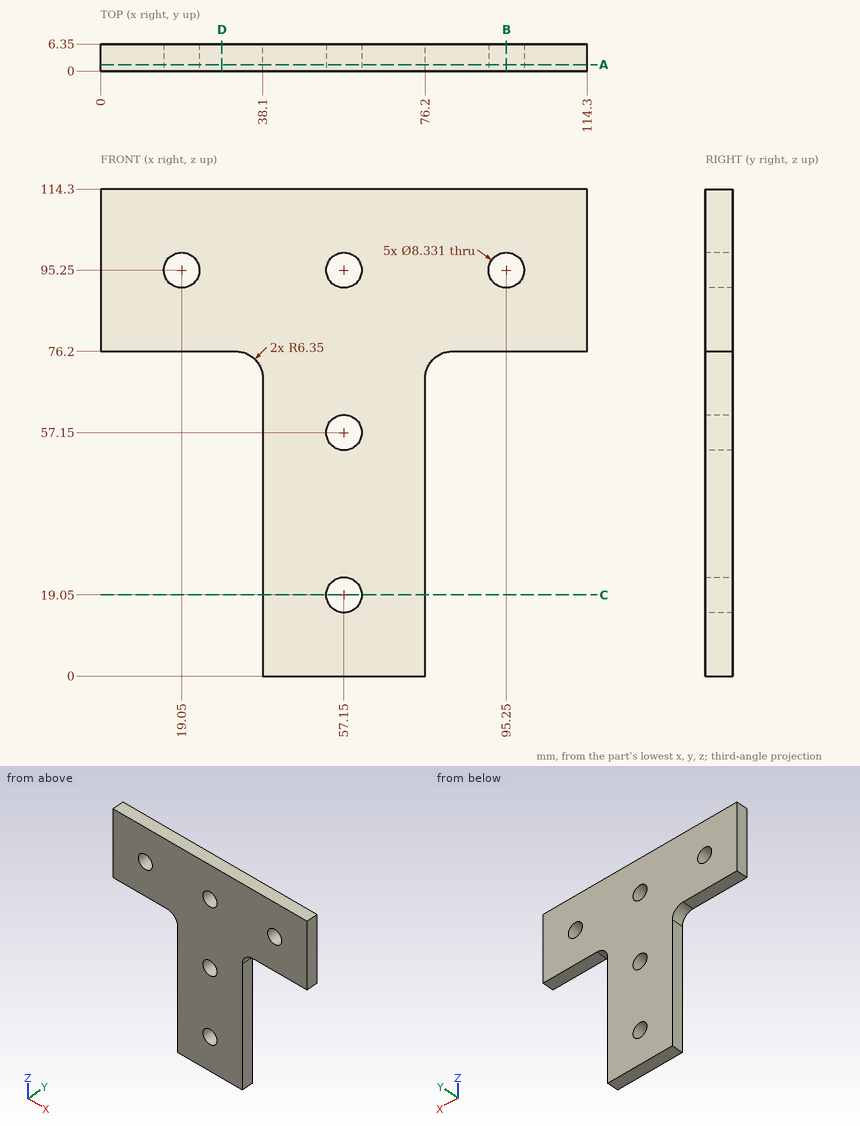
Geometry: see drawing. Coordinates: mm, zero at the bounding-box minimum. Give positions to 0.01 mm unless a question says otherwise; leave off trailing zeros. Order: outer loops, then holes, each group sorted by start corner. A loop starts at its lowest first (then second) coordinate and runs counter-clockwise, first axis right, second up. Notation, with made-up numbers: M 85,68 L 125,68 A36 cw 125,107 Z; hole C -8.5,88.5 d3. An arc over 180 degrees is marked long. Answer as a JSON object with one key per item and string values.
1. First-contact query: P1, Ø6.5, axis at x = 57.15, z = 19.05, coming from the +Y side; P2, Ø3, axis at y = 4.5, z = 51.5, coming from the +X side; P3, Ø3, axis at x = 74, y = 5.5, coming from the -Z side; P4, Ø2, axis at y = 1, z = 38.5, coming from the -X side. Flat tips, straight axial feed; report the tip coordinate or a pass-through.
Result sheet:
{"P1": "through", "P2": "x = 76.2", "P3": "z = 0", "P4": "x = 38.1"}
2. Cut plane C-C, the plane z = 19.05. Output: boundary loops of the cut face in (x, y), and give its area (3 significant figures).
Result sheet:
{"outline": "M 38.1,0 L 52.98,0 L 52.98,6.35 L 38.1,6.35 Z; M 61.32,0 L 76.2,0 L 76.2,6.35 L 61.32,6.35 Z", "area": "189 mm²"}
3. Cut plane B-B, the plane x = 95.25. Output: boundary loops of the cut face in (y, z).
Result sheet:
{"outline": "M 0,76.2 L 6.35,76.2 L 6.35,91.08 L 0,91.08 Z; M 0,99.42 L 6.35,99.42 L 6.35,114.3 L 0,114.3 Z"}
4. Cut plane D-D, the plane x = 28.5. Output: boundary loops of the cut face in (y, z), and give its area (3 significant figures).
Result sheet:
{"outline": "M 0,76.2 L 6.35,76.2 L 6.35,114.3 L 0,114.3 Z", "area": "242 mm²"}
5. Ray query, line 1 (X direction, y = 4, z = 95.25); line 2 (X direction, y = 5.25, z = 57.15); line 3 (X direction, y = 3, z = 12). Return the intervals inside material, ascending. Write a range as [from, to].
Result sheet:
{"line 1": "[0, 14.88], [23.22, 52.98], [61.32, 91.08], [99.42, 114.3]", "line 2": "[38.1, 52.98], [61.32, 76.2]", "line 3": "[38.1, 76.2]"}
6. Cut plane A-A, the plane y = 1.5. Output: boundary loops of the cut face in (x, z), and give its area (3 significant figures).
Result sheet:
{"outline": "M 0,76.2 L 31.75,76.2 A6.35 cw 38.1,69.85 L 38.1,0 L 76.2,0 L 76.2,69.85 A6.35 cw 82.55,76.2 L 114.3,76.2 L 114.3,114.3 L 0,114.3 Z; hole C 19.05,95.25 d8.33; hole C 57.15,19.05 d8.33; hole C 57.15,57.15 d8.33; hole C 57.15,95.25 d8.33; hole C 95.25,95.25 d8.33", "area": "7,000 mm²"}
